Check sheet for the drawn part. Datum: minimum x, y, z corner. Units: mm. Coordinates: 2 decimals unless noted, no trailing zeros. Write each loop counter-clockwise with the first axis right and the second up, starting at its lowest first coordinate (ties: lowest second). Pieces come first, ordered by that corner, then holes. Notation, with made-up numbers: (-19.75, 82) -> (17.25, 82) arc R26 ccw to (17.25, 120) -> close; hole circle Ø8 at (-33, 88.5). An arc over 180 degrees is marked (long way). Answer in a Markdown table with one row per item. Add a question column.
1. Cross-section at C-C on x = 30. Record the cut outline in (y, z) (3 decimals).
2. Cross-section at A-A on y = 39.37. Record the cut outline in (x, z) (3 decimals).
3. Cross-section at B-B on z = 2. Record the cut outline in (x, y), and give its area (3 significant figures).
4. Cross-section at D-D on y = 19.5. Record the cut outline in (x, z) (3 decimals), and give its area (3 significant figures).
5. Depth check by flat-ended pin: P1, Ø4.5, axis at x = 83.82, y = 113.03, coming from the -Z side. Enter the tip coordinate at first touch or a pass-through.
6. Scan lines: L1, parallel to Y at x = 160, z = 1.2; L2, parallel to X at y = 130.5, z = 2.05. Record each from-to range of solid material in increasing order. Write a range as from..to.
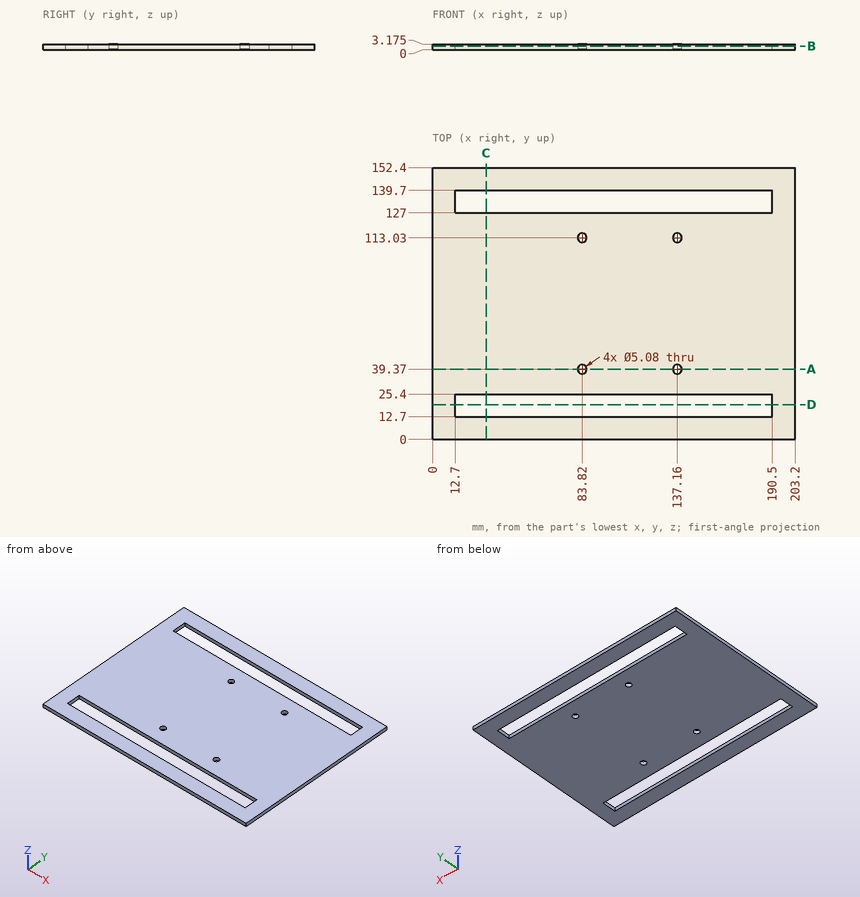
Results found:
| question | item | result |
|---|---|---|
| 1 | outline | (0, 0) -> (12.7, 0) -> (12.7, 3.175) -> (0, 3.175) -> close; (25.4, 0) -> (127, 0) -> (127, 3.175) -> (25.4, 3.175) -> close; (139.7, 0) -> (152.4, 0) -> (152.4, 3.175) -> (139.7, 3.175) -> close |
| 2 | outline | (0, 0) -> (81.28, 0) -> (81.28, 3.175) -> (0, 3.175) -> close; (86.36, 0) -> (134.62, 0) -> (134.62, 3.175) -> (86.36, 3.175) -> close; (139.7, 0) -> (203.2, 0) -> (203.2, 3.175) -> (139.7, 3.175) -> close |
| 3 | outline | (0, 0) -> (203.2, 0) -> (203.2, 152.4) -> (0, 152.4) -> close; hole (12.7, 12.7) -> (190.5, 12.7) -> (190.5, 25.4) -> (12.7, 25.4) -> close; hole (12.7, 127) -> (190.5, 127) -> (190.5, 139.7) -> (12.7, 139.7) -> close; hole circle Ø5.08 at (83.82, 39.37); hole circle Ø5.08 at (83.82, 113.03); hole circle Ø5.08 at (137.16, 39.37); hole circle Ø5.08 at (137.16, 113.03) |
| 3 | area | 26,400 mm^2 |
| 4 | outline | (0, 0) -> (12.7, 0) -> (12.7, 3.175) -> (0, 3.175) -> close; (190.5, 0) -> (203.2, 0) -> (203.2, 3.175) -> (190.5, 3.175) -> close |
| 4 | area | 80.6 mm^2 |
| 5 | P1 | passes through |
| 6 | L1 | y = 0..12.7, 25.4..127, 139.7..152.4 |
| 6 | L2 | x = 0..12.7, 190.5..203.2 |
